```python
from build123d import *

# Parameters (mm, degrees)
SKETCH1_W           = 15
SKETCH1_H           = 4
BOSS_EXTRUDE1_DEPTH = 300
CUT_EXTRUDE1_DEPTH  = 301.401398133
CUT_EXTRUDE2_DEPTH  = 2


with BuildPart() as part:
    # Sketch1 → Boss-Extrude1 (new body)
    with BuildSketch(Plane(origin=(0, 0, 0), x_dir=(0, 0, -1), z_dir=(1, 0, 0))):
        with Locations((7.5, -2)):
            Rectangle(SKETCH1_W, SKETCH1_H)
    extrude(amount=BOSS_EXTRUDE1_DEPTH)

    # Sketch3 → Cut-Extrude1 (cut, through all)
    with BuildSketch(Plane(origin=(0, 0, 0), x_dir=(1, 0, 0), z_dir=(0, 1, 0))):
        with BuildLine():
            Line((10, 9.5), (26, 9.5))
            ThreePointArc((26, 9.5), (28, 7.5), (26, 5.5))
            Line((26, 5.5), (10, 5.5))
            ThreePointArc((10, 5.5), (8, 7.5), (10, 9.5))
        make_face()
        with BuildLine():
            Line((266, 9.5), (282, 9.5))
            ThreePointArc((282, 9.5), (284, 7.5), (282, 5.5))
            Line((282, 5.5), (266, 5.5))
            ThreePointArc((266, 5.5), (264, 7.5), (266, 9.5))
        make_face()
    extrude(amount=-CUT_EXTRUDE1_DEPTH, mode=Mode.SUBTRACT)

    # Sketch4 → Cut-Extrude2 (cut)
    with BuildSketch(Plane(origin=(0, 0, 0), x_dir=(1, 0, 0), z_dir=(0, 1, 0))):
        with BuildLine():
            Line((10, 11.6), (26, 11.6))
            ThreePointArc((26, 11.6), (30.1, 7.5), (26, 3.4))
            Line((26, 3.4), (10, 3.4))
            ThreePointArc((10, 3.4), (5.9, 7.5), (10, 11.6))
        make_face()
        with BuildLine():
            Line((266, 11.6), (282, 11.6))
            ThreePointArc((282, 11.6), (286.1, 7.5), (282, 3.4))
            Line((282, 3.4), (266, 3.4))
            ThreePointArc((266, 3.4), (261.9, 7.5), (266, 11.6))
        make_face()
    extrude(amount=-CUT_EXTRUDE2_DEPTH, mode=Mode.SUBTRACT)


solid = part.part
```
Design review of the part built by this model. Coordinates are the model's own, in mm. A direction names the side the tool comes from. Round coordinates to 2 decimals unless told otherwise and drop trailing zeros. Order: outer loops, then holes, each group sorted by start corner. A loop starts at its lowest first (then second) coordinate and runs counter-clockwise, first axis right, second up. Notation, with made-up numbers: (66.5, 10.5) - (95.5, 10.5) arc R12 ccw to (95.5, 21.5) - close; hole circle Ø1 at (-30.5, 52). An arc over 180 degrees is marked (long way). Return JSON: item names as keys, results as strings.
Q1. Wall thickness on L1, parallel to Z at x = 277, y = -1; L2, parallel to Y at x = 27.5, z = -5.75; L3, parallel to X at y = -0.5, z = -6.75: over which ranges is each line inside the solid? List them lowest first. Write a range as [from, to].
Computed values:
{"L1": "z = [-15, -11.6], [-3.4, 0]", "L2": "y = [-4, -2]", "L3": "x = [0, 5.97], [30.03, 261.97], [286.03, 300]"}
Q2. Consider section A-A on y = -3.4. Write out the cut boundary in (x, z).
Computed values:
{"outline": "(0, -15) - (300, -15) - (300, 0) - (0, 0) - close; hole (10, -9.5) - (26, -9.5) arc R2 ccw to (26, -5.5) - (10, -5.5) arc R2 ccw to start; hole (266, -9.5) - (282, -9.5) arc R2 ccw to (282, -5.5) - (266, -5.5) arc R2 ccw to start"}
Q3. The part is to be moulded in two halves that separate along X. For faces 1 (the flat face through (148, 0, -7)), 2 (the flat face through (274, -2, -5)), say which applies: pulls with the +X half, pulls with the -X half, needs draft (parallel to the pull), parting line crosses it, or undercut.
Computed values:
{"face 1": "needs draft", "face 2": "undercut"}
Q4. Machinability: for faces 3 (the flat face through (18, -2, -5)), 4 (the flat face through (148, -4, -7)), which of the approach directions +Z, -Z, +X, -X, +Y, -Y give a long, thin tool a straight path to every point of the face, cutting with its end or side? Answer none if there is none.
Computed values:
{"face 3": "+Y", "face 4": "+Z, -Z, +X, -X, -Y"}
Q5. For pin 1 Ø2.5 at (x, z) = (269, -6.5) entering from +Y, flat-tipped, find the tip position at first contact; note if it passes through.
Computed values:
{"pin 1": "stops at y = -2"}
